Input: dimensioned drawing with shaded views. Units: mm. Origin: part minimum x, y, z. A direction names the side the tool comes from. Round coordinates to 2 decimals unless told otherwise and drop trailing zeros. Loops run counter-clockwise (first coordinate to the right, second up) from the corner with the lowest first, then second, coordinate; pieces in that order, holes last.
1) Section A-A, the plane x = 374.5. Return loops of the section in (y, z).
2) Access query for the marked faces 1, 2 and 3. Directions: +Z, -Z, +X, -X, +Y, -Y. A direction counts if a zero-diameter tool reaches every point of the face in a straight line with its end or side. Return the directions, or none.
3) Section D-D, the plane x = 883. Return loops of the section in (y, z), and give its area (3 significant figures).
4) Ray query, line 1 along X through (y, z) = (319, 377.5); line 2 along Z through (x, y) = (247.5, 362); line 3 along X through (y, z) = (451.5, 72) (1 decimal). Return the intervals inside material, ascending.
5) Section B-B, the plane y = 383. Return loops of the section in (x, z) (1 decimal), and give its area (3 significant figures).
6) First-contact query: pin 1 (5 mm diameter, centred on y = 161, z = 231.5, fed in from -X) (1 decimal); pin 2 (6 mm diameter, centred on x = 394, y = 159.5, fed in from -Z); pin 3 (2 mm diameter, centred on y = 455.5, z = 403, fed in from +X). Flat tips, straight axial feed; report the tip coordinate or a pass-through.
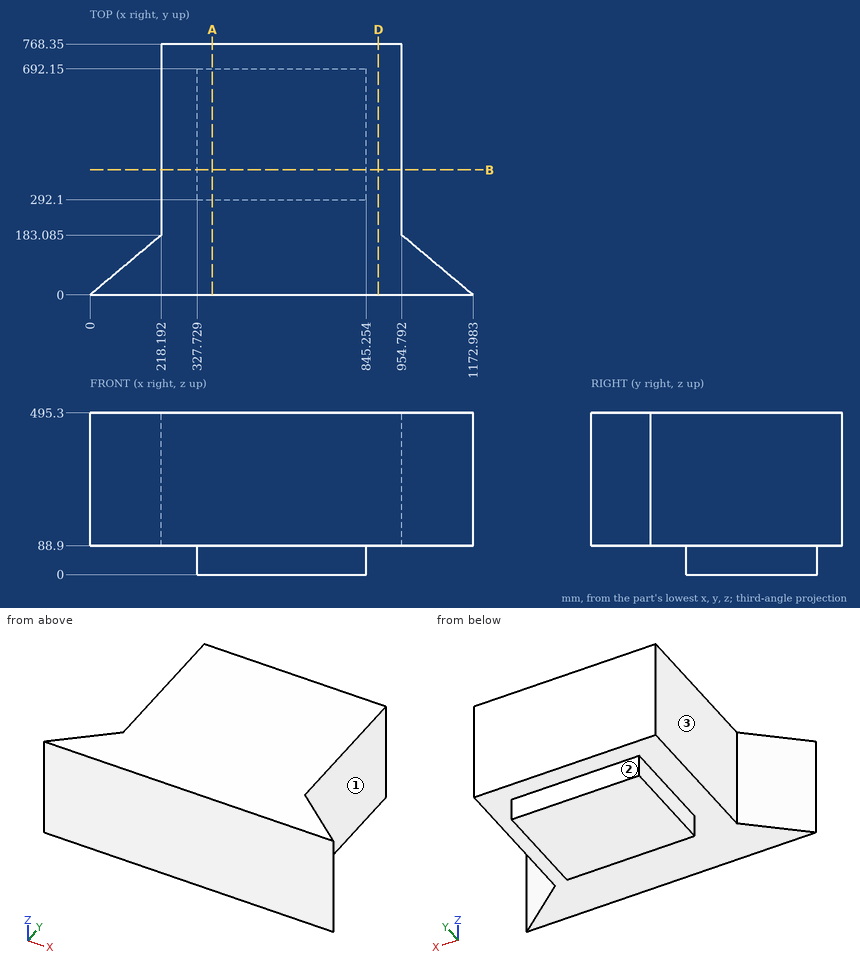
Final values:
1. outline: (0, 88.9) - (292.1, 88.9) - (292.1, 0) - (692.15, 0) - (692.15, 88.9) - (768.35, 88.9) - (768.35, 495.3) - (0, 495.3) - close
2. face 1: +Z, -Z, +X, +Y
2. face 2: -Z, +X, -X, +Y
2. face 3: +Z, -Z, -X, +Y
3. outline: (0, 88.9) - (768.35, 88.9) - (768.35, 495.3) - (0, 495.3) - close
3. area: 312,000 mm2
4. line 1: x = 218.19 to 954.79
4. line 2: z = 88.9 to 495.3
4. line 3: x = 327.7 to 845.3
5. outline: (218.2, 88.9) - (327.7, 88.9) - (327.7, 0) - (845.3, 0) - (845.3, 88.9) - (954.8, 88.9) - (954.8, 495.3) - (218.2, 495.3) - close
5. area: 345,000 mm2
6. pin 1: stops at x = 188.9
6. pin 2: stops at z = 88.9
6. pin 3: stops at x = 954.79
